Input: part model. Units: mm. Frame: model coordinates. Face numbers are marked on the shaded views. A direction names the side the tool comes from. Coordinates: 2 decimals unless noted, no trailing zeros. Write each loop counter-clockwise with the first axis right and the second up, starting at its lowest first coordinate (ties: lowest second). Pieces come first, ordered by that corner, then holes. Notation, with made-up numbers: (38, -36.75) - (65, -36.75) arc R30 cw to (65, -13.75) - close; hole circle Ø6 at (10.5, -1). An arc over 180 degrees is marked (long way). Put each result on its own line as item: value. Start each with the question number.
1. Pull-direction query (Y, two-part tool) for the marked faces 1, 2 and 3; classes: released by +Y, released by -Y, zero draft, split by the parting line, or undercut.
2. Cut plane B-B, the plane z = 18. Return loops of the section in (x, y), and give its area (3 significant figures).
3. Line query: line 1 (Y direction, x = 4.5, z = 11); line 2 (X direction, y = 5.5, z = 2); line 3 (X direction, y = 7.5, z = 4). Output: solid intervals per line, ascending.
4. Cut plane D-D, the plane z = 4.25. Return loops of the section in (x, y), and give its area (3 significant figures).
5. Cut plane A-A, the plane x = 27. Return loops of the section in (y, z), and give its area (3 significant figures).
6. Access query for the marked faces 4, 5 and 6. Directions: +Z, -Z, +X, -X, +Y, -Y. A direction counts if a zero-diameter tool reaches every point of the face in a straight line with its end or side. Return the directions, or none.
7. Pin query (flat end, axial travel): pin 1 (6 mm diameter, centred on x = 11, y = 4.5, fed in from +Z); pin 2 (6 mm diameter, centred on x = 9, y = 6, fed in from +Z). Return the tip coordinate at first contact, or that it passes through.
8. Cut plane C-C, the plane y = 8.5. Return loops of the section in (x, z).
from build123d import *

# Parameters (mm, degrees)
F1_DEPTH = 20
F2_W     = 25
F2_H     = 10
F3_DEPTH = 10
F4_W     = 10
F4_H     = 5
F4_H_2   = 2.5
F5_DEPTH = 5


with BuildPart() as f1:
    # F0 (on Front) → F1 (new body)
    with BuildSketch(Plane.XZ):
        Polygon((30, 5), (0, 20), (0, 0), (30, 0), align=None)
    extrude(amount=-F1_DEPTH)

    # F2 (on face) → F3 (cut)
    with BuildSketch(Plane(origin=(8, 0, 16), x_dir=(0.894427191, 0, -0.4472135955), z_dir=(0.4472135955, 0, 0.894427191))):
        with Locations((3.55572809, 10)):
            Rectangle(F2_W, F2_H)
    extrude(amount=-F3_DEPTH, mode=Mode.SUBTRACT)

    # F4 (on face) → F5 (cut)
    with BuildSketch(Plane.YZ.offset(30)):
        with Locations((10, 2.5)):
            Rectangle(F4_W, F4_H)
        with Locations((10, 6.25)):
            Rectangle(F4_W, F4_H_2)
    extrude(amount=-F5_DEPTH, mode=Mode.SUBTRACT)


solid = f1.part
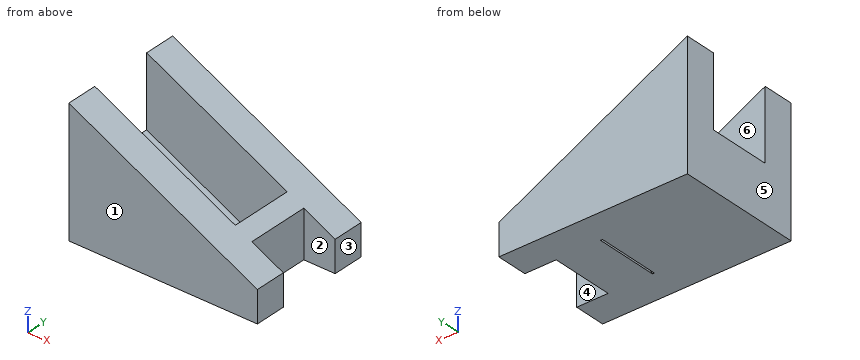
Report:
1. face 1: released by -Y
1. face 2: undercut
1. face 3: zero draft
2. outline: (0, 0) - (4, 0) - (4, 5) - (0, 5) - close; (0, 15) - (4, 15) - (4, 20) - (0, 20) - close
2. area: 40.0 mm^2
3. line 1: y = 0 to 5, 15 to 20
3. line 2: x = 0 to 13.64, 18.95 to 25
3. line 3: x = 0 to 9.64, 19.95 to 25
4. outline: (0, 0) - (30, 0) - (30, 5) - (25, 5) - (25, 15) - (30, 15) - (30, 20) - (0, 20) - close; hole (9.14, 5) - (20.08, 5) - (20.08, 15) - (9.14, 15) - close
4. area: 441 mm^2
5. outline: (0, 0) - (5, 0) - (5, 6.5) - (0, 6.5) - close; (15, 0) - (20, 0) - (20, 6.5) - (15, 6.5) - close
5. area: 65.0 mm^2
6. face 4: +Z, -Z, +X
6. face 5: +Z, -Z, -X, +Y, -Y
6. face 6: +Z
7. pin 1: stops at z = 16
7. pin 2: stops at z = 16.91
8. outline: (0, 0) - (17.64, 0) - (0, 8.82) - close; (17.95, 0) - (25, 0) - (25, 7.5) - (22.36, 8.82) - close
